```python
from build123d import *

# Parameters (mm, degrees)
F0_W      = 29
F0_H      = 16.5
F1_DEPTH  = 38.5
F2_T      = -2
F3_DEPTH  = 2.5
F4_SIZE   = 2
F5_SIZE   = 2
F6_SIZE   = 0.99999
F8_DEPTH  = 16.501
F9_W      = 7.54
F9_H      = 7.25
F9_R      = 1.1
F10_DEPTH = 6.35
F13_W     = 5.538
F13_H     = 4.583
F11_W     = 5.533
F11_H     = 5.533


# Not quite as in the source:
# - a fillet or chamfer is up to 0.001 mm smaller than in the source, because OpenCascade refuses the exact size


with BuildPart() as f1:
    # F0 (on Top) → F1 (new body)
    with BuildSketch(Plane.XY):
        with Locations((14.5, 8.25)):
            Rectangle(F0_W, F0_H)
    extrude(amount=F1_DEPTH)

    # F2
    f2_openings = [f1.faces().sort_by_distance(p)[0] for p in [
        (14.5, 8.25, 38.5),
    ]]
    offset(amount=F2_T, openings=f2_openings)

    # F3 (add): a face of the model
    f3_faces = [f1.faces().sort_by_distance(p)[0] for p in [
        (14.5, 8.25, 2),
    ]]
    extrude(f3_faces, amount=F3_DEPTH)

    # F4
    f4_edges = [f1.edges().sort_by_distance(p)[0] for p in [
        (29, 0, 19.25),
        (29, 16.5, 19.25),
        (0, 0, 19.25),
        (0, 16.5, 19.25),
    ]]
    chamfer(f4_edges, length=F4_SIZE)

    # F5
    f5_edges = [f1.edges().sort_by_distance(p)[0] for p in [
        (0, 8.25, 0),
        (1, 15.5, 0),
        (1, 1, 0),
        (14.5, 16.5, 0),
        (14.5, 0, 0),
        (28, 15.5, 0),
        (28, 1, 0),
        (29, 8.25, 0),
    ]]
    chamfer(f5_edges, length=F5_SIZE)

    # F6 (size 1 in the source; OpenCascade refuses exactly that, so slightly less here)
    f6_edges = [f1.edges().sort_by_distance(p)[0] for p in [
        (14.5, 16.5, 38.5),
        (0, 8.25, 38.5),
        (14.5, 0, 38.5),
        (29, 8.25, 38.5),
    ]]
    chamfer(f6_edges, length=F6_SIZE)

    # F7 (on face) → F8 (cut, through all)
    with BuildSketch(Plane.XZ):
        Polygon((12.635, 12.834), (6.464, 8.667), (6.464, 4.94), (23.536, 4.94), (23.536, 8.667), (17.365, 12.834), align=None)
    extrude(amount=-F8_DEPTH, mode=Mode.SUBTRACT)

    # F9 (on face) → F10 (join)
    with BuildSketch(Plane.YZ.offset(29)):
        with Locations((8.25, 7.875)):
            Rectangle(F9_W, F9_H)
        with Locations((8.25, 9)):
            Circle(F9_R, mode=Mode.SUBTRACT)
    extrude(amount=-F10_DEPTH)

    # F13 (on offset) → F14 section 0
    with BuildSketch(Plane.YZ.offset(24.55)):
        with Locations((8.258, 8.5135)):
            Rectangle(F13_W, F13_H)
    # F11 (on face) → F14 section 1
    with BuildSketch(Plane.YZ.offset(29)):
        with Locations((8.2475, 8.0385)):
            Rectangle(F11_W, F11_H)
    loft(mode=Mode.SUBTRACT)


solid = f1.part
```
Verification items for the finished model (mm, model axes). A direction names the side the tool comes from. Give positions to 0.01 mm unless a question says otherwise; leave off trailing zeros. Order: outer loops, then holes, each group sorted by start corner. A loop starts at its lowest first (then second) coordinate and runs counter-clockwise, first axis right, second up. Notation, with made-up numbers: (21, 63.25) -> (80, 63.25) arc R11 cw to (80, 79.25) -> close; hole circle Ø8 at (26, -15). An arc over 180 degrees is marked (long way). One line per item, written item: value.
(1) Gauge pin test, flat ends, axial feed: pin 1 (1.3 mm diameter, centred on x = 25.5, y = 8, fed in from +Z); pin 2 (6 mm diameter, centred on x = 15.5, y = 8, fed in from +Z); pin 3 (0.6 mm diameter, centred on y = 15, z = 7, fed in from +X). Record the tip position at first contact, or that the pin passes through.
Final values:
pin 1: z = 11.5
pin 2: z = 4.5
pin 3: x = 28.8
(2) Sectioned sample at B-B on z = 27.5. Record the cut outline in (x, y).
Final values:
outline: (0, 2) -> (2, 0) -> (27, 0) -> (29, 2) -> (29, 14.5) -> (27, 16.5) -> (2, 16.5) -> (0, 14.5) -> close; hole (2, 2) -> (27, 2) -> (27, 14.5) -> (2, 14.5) -> close
(3) Scan lines: line 1 along Y through (x, z) = (25, 9); line 2 along X through (y, z) = (6.75, 19.5); line 3 along Y through (x, z) = (13.25, 32). Record each from-to range of solid material in increasing order. Write a range as [from, to].
Final values:
line 1: [0, 2], [4.48, 5.49], [11.03, 12.02], [14.5, 16.5]
line 2: [0, 2], [27, 29]
line 3: [0, 2], [14.5, 16.5]
(4) Sectioned sample at D-D on x = 10. Record the cut outline in (y, z), then the cut area to 3 significant figures.
Final values:
outline: (0, 2) -> (2, 0) -> (14.5, 0) -> (16.5, 2) -> (16.5, 4.94) -> (14.5, 4.94) -> (14.5, 4.5) -> (2, 4.5) -> (2, 4.94) -> (0, 4.94) -> close; (0, 11.05) -> (2, 11.05) -> (2, 38.5) -> (1, 38.5) -> (0, 37.5) -> close; (14.5, 11.05) -> (16.5, 11.05) -> (16.5, 37.5) -> (15.5, 38.5) -> (14.5, 38.5) -> close
area: 181 mm^2
(5) Sectioned sample at A-A on x = 18.75. Record the cut outline in (y, z), then the cut area to 3 significant figures.
Final values:
outline: (0, 2) -> (2, 0) -> (14.5, 0) -> (16.5, 2) -> (16.5, 4.94) -> (14.5, 4.94) -> (14.5, 4.5) -> (2, 4.5) -> (2, 4.94) -> (0, 4.94) -> close; (0, 11.9) -> (2, 11.9) -> (2, 38.5) -> (1, 38.5) -> (0, 37.5) -> close; (14.5, 11.9) -> (16.5, 11.9) -> (16.5, 37.5) -> (15.5, 38.5) -> (14.5, 38.5) -> close
area: 177 mm^2
(6) Sectioned sample at C-C on y = 3.25. Record the cut outline in (x, z), then the cut area to 4 significant figures.
Final values:
outline: (0, 2) -> (2, 0) -> (27, 0) -> (29, 2) -> (29, 37.5) -> (28, 38.5) -> (27, 38.5) -> (27, 4.5) -> (2, 4.5) -> (2, 38.5) -> (1, 38.5) -> (0, 37.5) -> close
area: 261.5 mm^2
(7) Tool access check on faces 5 (the face through (23.613, 9.266, 8.579)), 6 (the face through (14, 2, 25)), 7 (the face through (6.464, 1, 7)). Record the directions out of +Z, -Z, +X, -X, +Y, -Y that give a thin tool (end or side, any length) a straight path to the whole face; none if there is none.
Final values:
face 5: +X
face 6: +Z
face 7: +Y, -Y
(8) Draft check along X on faces 1 (the face through (1.55, 1.57, 1.21)), 2 (the face through (14, 1, 1)), 3 (the face through (27.45, 14.93, 1.21)), 4 (the face through (25, 8, 11.5)). Enter one of: pulls with the +X half, pulls with the -X half, needs draft (parallel to the pull), parting line crosses it, or undercut.
Final values:
face 1: pulls with the -X half
face 2: needs draft
face 3: pulls with the +X half
face 4: undercut
